```python
from build123d import *

# Parameters (mm, degrees)
BOSS_EXTRUDE1_DEPTH = 3
CUT_EXTRUDE1_DEPTH  = 10
CIRPATTERN1_COUNT   = 6
BOSS_EXTRUDE2_DEPTH = 10
SKETCH6_R           = 32
CUT_EXTRUDE2_DEPTH  = 3.5
SKETCH7_R           = 20
SKETCH7_R_2         = 11
CUT_EXTRUDE4_DEPTH  = 5.5
BOSS_EXTRUDE3_DEPTH = 5.5
CIRPATTERN2_COUNT   = 16
SKETCH10_R          = 19
BOSS_EXTRUDE4_DEPTH = 4.5
SKETCH11_R          = 18
CUT_EXTRUDE5_DEPTH  = 25.5
SKETCH12_R          = 8
SKETCH12_R_2        = 7
BOSS_EXTRUDE5_DEPTH = 5
SKETCH13_R          = 7
CUT_EXTRUDE6_DEPTH  = 23
SKETCH14_R          = 2
CUT_EXTRUDE9_DEPTH  = 6


with BuildPart() as part:
    # Sketch2 → Revolve2 (revolve)
    with BuildSketch(Plane.XY):
        Polygon((0, 0), (0, 33), (-7, 32.210806874), (-7, 24.5371762), (-15, 24.5371762), (-15, 35), (-17.5, 35), (-17.5, 20), (-40, 20), (-40, 0), align=None)
    revolve(axis=Axis((0, 0, 0), (-1, 0, 0)))

    # Sketch3 → Boss-Extrude1 (add)
    with BuildSketch(Plane.ZY.offset(17.5)):
        with BuildLine():
            Line((-1.119688757, 19.96863283), (-1.119688757, 31.952311667))
            Line((-1.119688757, 31.952311667), (1.380311243, 31.952311667))
            Line((1.380311243, 31.952311667), (1.380311243, 19.952311667))
            ThreePointArc((1.380311243, 19.952311667), (0.130566516, 19.999573805), (-1.119688757, 19.96863283))
        make_face()
    boss_extrude1 = extrude(amount=BOSS_EXTRUDE1_DEPTH)

    # Sketch4 → Cut-Extrude1 (cut)
    with BuildSketch(Plane.XY.offset(1.380311243)):
        Polygon((-20.5, 19.952311667), (-17.5, 31.952311667), (-20.5, 31.952311667), align=None)
    cut_extrude1 = extrude(amount=-CUT_EXTRUDE1_DEPTH, mode=Mode.SUBTRACT)

    # CirPattern1: Boss-Extrude1, Cut-Extrude1 ×6 about axis
    cirpattern1_axis = Axis((0, 0, 0), (1, 0, 0))
    for i in range(1, CIRPATTERN1_COUNT):
        add(boss_extrude1.rotate(cirpattern1_axis, i * 360 / CIRPATTERN1_COUNT))
        add(cut_extrude1.rotate(cirpattern1_axis, i * 360 / CIRPATTERN1_COUNT), mode=Mode.SUBTRACT)

    # Sketch5 → Boss-Extrude2 (add)
    with BuildSketch(Plane.ZY.offset(17.5)):
        with BuildLine():
            Line((0.341434911, -18.344937093), (15.591504627, -9.672552828))
            Line((15.591504627, -9.672552828), (22.828663164, -22.398830732))
            ThreePointArc((22.828663164, -22.398830732), (15.809898035, -27.801125951), (7.578593448, -31.071214997))
            Line((7.578593448, -31.071214997), (0.341434911, -18.344937093))
        make_face()
        with BuildLine():
            Line((2.659566405, -18.98232738), (14.95411434, -11.990684322))
            Line((14.95411434, -11.990684322), (20.702890868, -22.099697042))
            ThreePointArc((20.702890868, -22.099697042), (14.969527432, -26.323365061), (8.408342933, -29.091340099))
            Line((8.408342933, -29.091340099), (2.659566405, -18.98232738))
        make_face(mode=Mode.SUBTRACT)
    extrude(amount=BOSS_EXTRUDE2_DEPTH)

    # Sketch6 → Cut-Extrude2 (cut)
    with BuildSketch(Plane(origin=(0, 0, 0), x_dir=(0, 0, -1), z_dir=(1, 0, 0))):
        Circle(SKETCH6_R)
    extrude(amount=-CUT_EXTRUDE2_DEPTH, mode=Mode.SUBTRACT)

    # Sketch7 → Cut-Extrude4 (cut)
    with BuildSketch(Plane(origin=(-3.5, 0, 0), x_dir=(0, 0, -1), z_dir=(1, 0, 0))):
        Circle(SKETCH7_R)
        Circle(SKETCH7_R_2, mode=Mode.SUBTRACT)
    extrude(amount=-CUT_EXTRUDE4_DEPTH, mode=Mode.SUBTRACT)

    # Sketch9 → Boss-Extrude3 (add)
    with BuildSketch(Plane(origin=(-9, 0, 0), x_dir=(0, 0, -1), z_dir=(1, 0, 0))):
        with BuildLine():
            Line((0.75, 10.60425024), (0.75, 20.365350298))
            ThreePointArc((0.75, 20.365350298), (0, 20.37915584), (-0.75, 20.365350298))
            Line((-0.75, 20.365350298), (-0.75, 10.60425024))
            ThreePointArc((-0.75, 10.60425024), (0, 10.630739539), (0.75, 10.60425024))
        make_face()
    boss_extrude3 = extrude(amount=BOSS_EXTRUDE3_DEPTH)

    # CirPattern2: Boss-Extrude3 ×16 about axis
    cirpattern2_axis = Axis((0, 0, 0), (1, 0, 0))
    for i in range(1, CIRPATTERN2_COUNT):
        add(boss_extrude3.rotate(cirpattern2_axis, i * 360 / CIRPATTERN2_COUNT))

    # Sketch10 → Boss-Extrude4 (add)
    with BuildSketch(Plane(origin=(-9, 0, 0), x_dir=(0, 0, -1), z_dir=(1, 0, 0))):
        Circle(SKETCH10_R)
    extrude(amount=BOSS_EXTRUDE4_DEPTH)

    # Sketch11 → Cut-Extrude5 (cut)
    with BuildSketch(Plane.ZY.offset(40)):
        Circle(SKETCH11_R)
    extrude(amount=-CUT_EXTRUDE5_DEPTH, mode=Mode.SUBTRACT)

    # Sketch12 → Boss-Extrude5 (add)
    with BuildSketch(Plane.ZY.offset(14.5)):
        Circle(SKETCH12_R)
        Circle(SKETCH12_R_2, mode=Mode.SUBTRACT)
    extrude(amount=BOSS_EXTRUDE5_DEPTH)

    # Sketch13 → Cut-Extrude6 (cut)
    with BuildSketch(Plane.ZY.offset(14.5)):
        Circle(SKETCH13_R)
    extrude(amount=-CUT_EXTRUDE6_DEPTH, mode=Mode.SUBTRACT)

    # Sketch14 → Cut-Extrude9 (cut)
    with BuildSketch(Plane(origin=(-15, 0, 0), x_dir=(0, 0, -1), z_dir=(1, 0, 0))):
        with Locations((-13.549564178, -23.82641175)):
            Circle(SKETCH14_R)
    extrude(amount=-CUT_EXTRUDE9_DEPTH, mode=Mode.SUBTRACT)


solid = part.part
```
Here's how the part is built. I have some questions about the finished solid (model axes, mm). A direction names the side the tool comes from. Round coordinates to 2 decimals unless told otherwise and drop trailing zeros. Loops run counter-clockwise (first coordinate to the right, second up) from the corner with the lowest first, then second, coordinate; pieces in that order, holes last.
1. For faces 1 (the face through (-19, -25, 1.12)), 2 (the face through (-9, -4, 19)), 3 (the face through (-18.644, 11.303, -21.816)), 4 (the face through (-16, -28, 21)), which set-ups out of +Z, -Z, +X, -X, +Y, -Y let a thin tool reach every point of the face, with its end or its side?
Answers:
face 1: -X, -Y
face 2: +X
face 3: -Z, -X
face 4: +X, -X
2. Suppose I cut it at B-B, the plane x = -28.5. Please give me the cut outline in (y, z).
Answers:
outline: circle Ø40 at (0, 0); hole circle Ø36 at (0, 0)
3. Suppose I cut it at A-A, the plane x = -21.5. Please give me the cut outline in (y, z).
Answers:
outline: (-31.07, 7.58) - (-19.96, 1.26) arc R20 ccw (long way) to (-11.29, 16.51) - (-22.4, 22.83) arc R31.98 ccw to start; hole (-29.09, 8.41) - (-19.76, 3.1) arc R20 cw to (-12.77, 15.4) - (-22.1, 20.7) arc R30.28 ccw to start; hole circle Ø36 at (0, 0)
4. Thinking about a two-plate mould opening in Y: for faces 5 (the face through (-22.43, -27.74, 15.92)), 6 (the face through (-4.23, -12.17, -11.11)), 7 (the face through (-19, 25, -1.12)), which applies, released by +Y, released by -Y, zero draft, split by the parting line, or undercut?
Answers:
face 5: released by -Y
face 6: undercut
face 7: zero draft
5. Suppose I cut it at C-C, the plane x = -11. Please give me the cut outline in (y, z), and give its area (3 significant figures).
Answers:
outline: circle Ø49.07 at (0, 0); hole circle Ø14 at (0, 0)
area: 1,740 mm2
6. If I drill on probe 1 along Y at (x, z) = (-7.5, 1); probe 2 along Y at (x, z) = (-22.75, 0); probe 3 along Y at (x, z) = (-21.5, 5), over which ranges is the centre line in solid material (lowest first)?
Answers:
probe 1: y = -24.52 to -19.97, -18.97 to -6.93, 6.93 to 18.97, 19.97 to 24.52
probe 2: y = -20 to -18, 18 to 20
probe 3: y = -26.54 to -23.1, -19.36 to -17.29, 17.29 to 19.36
7. Will these pins go through, and if not, where does the flat tip stop? pin 1 (2.5 mm diameter, centred on y = 15, z = -8, fed in from +X); pin 2 (1 mm diameter, centred on y = -26, z = 20.5, fed in from +X); pin 3 (8 mm diameter, centred on y = -12, z = -7, fed in from -X); pin 4 (5 mm diameter, centred on x = -22, y = 0.5, fed in from -Z).
Answers:
pin 1: stops at x = -3.5
pin 2: stops at x = 0
pin 3: stops at x = -14.5
pin 4: stops at z = -20
